Autodesk Inventor part; units mm, degrees
ref_plane "YZ Plane" through (0, 0, 0) normal (1, 0, 0) x (0, 1, 0)
ref_plane "XZ Plane" through (0, 0, 0) normal (0, 1, 0) x (-1, 0, 0)
ref_plane "XY Plane" through (0, 0, 0) normal (0, 0, 1) x (1, 0, 0)
sketch "Sketch1" plane through (0, 0, 0) normal (0, 1, 0) x (-1, 0, 0)
  circle A0 centre (0, 0) radius 304.8
  dimension "d0" = 609.6
extrude "Extrusion1" add sketch "Sketch1" along normal blind 914.4
fillet "Fillet1" radius 254 1 edges at (304.8, 914.4, 0)
fillet "Fillet2" radius 127 1 edges at (304.8, 0, 0)
properties part number "Pool Filter"
For this review, take the finished solid that the model builds, in its own axes (mm). Coordinates: 2 decimals unless noted, no trailing zeros. Order: outer loops, then holes, each group sorted by start corner. A loop starts at its lowest first (then second) coordinate and runs counter-clockwise, first axis right, second up. Notation, with made-up numbers: (19, 9) -> (47, 9) arc R25 ccw to (47, 39) -> close; hole circle Ø2 at (-14, -23.5). An arc over 180 degrees is marked (long way). Return JSON: item names as keys, results as strings.
1. For line 1 (Z direction, x = 8, y = 347) (3 decimals); line 2 (Z direction, x = -9, y = 257.5); line 3 (Y direction, x = -29, z = 237.5), list the stretches that pass through material, from the lowest coordinate up. Write a range as from..to.
Answer block:
{"line 1": "-304.695..304.695", "line 2": "-304.67..304.67", "line 3": "15.86..830.69"}
2. For pin 1 Ø8 at (x, z) = (-99.5, -209.5) entering from -Y; pin 2 Ø10 at (x, y) = (36, 432.5) entering from -Z; pin 3 Ø5 at (x, y) = (164.5, 266) entering from -Z, all flat-tipped, find the tip position at first contact; note any pin that passes through.
Answer block:
{"pin 1": "y = 10.31", "pin 2": "z = -303.22", "pin 3": "z = -258.18"}
3. We need section A-A on y = 191.5. Write out the cut boundary in (x, z), and give its area (3 significant figures).
Answer block:
{"outline": "circle Ø609.6 at (0, 0)", "area": "292,000 mm²"}
